The listing builds one solid part. Answer for the finished solid, in the listing's coordinates (mm). A direction names the side the tool comes from. Give positions to 0.01 mm unless a question says otherwise; leave off trailing zeros. Loops run counter-clockwise (first coordinate to the right, second up) from the corner with the lowest first, then second, coordinate; pieces in that order, holes last. Notation, with made-up numbers: M 57.25,19.25 L 68.25,19.25 A28 cw 68.25,57.25 Z; hole C 20.25,36.25 d7. An arc over 180 degrees is marked long. One line per item, written item: value. Start each with the question number.
Q1. A cutting plane is placed at D-D, the plane x = 47.5. Determine the outline of the cut face in (y, z), and give its area (3 significant figures).
Q2. Flat-ended cylindrical pins translate along their axes: pin 1 (8 mm diameter, centred on x = 54.5, y = 20, fed in from +Z); pin 2 (5 mm diameter, centred on x = 47.5, y = 15, fed in from +Z). Find the tip coordinate at first contact, or state that the pin passes through.
Q3. The mould has two halves that part along Y. Classify faces 1 (the flat face through (4.5, 5.7, 6)), 2 (the flat face through (32, 0, 1)), 3 (the cylindrical face through (4.109, 45.974, 4.479)), 4 (the cylindrical face through (59.763, 43.676, 2.958)): +Y half, -Y half, draft (parallel to the pull), parting line (faces both ways), or undercut.
Q4. A cutting plane is placed at A-A, the plane z = 5. Determine the outline of the cut face in (x, y).
Q5. A cutting plane is placed at C-C, the plane y = 43. Determine the outline of the cut face in (x, z).
Q6. For faces 5 (the cylindrical face through (58.29, 45.03, 4.48)), 6 (the flat face through (32, 25, 0)), determine the directions among +Z, -Z, +X, -X, +Y, -Y from which every point of the face is accessible in a straight line to the end or side of a thin tool.
Q7. A cutting plane is placed at B-B, the plane x = 4.5. Determine the outline of the cut face in (y, z).
Q8. Consider L1, parallel to Y at x = 60.5, z = 1.3; L2, parallel to Y at x = 4.5, z = 3.05; L3, parallel to Z at x = 36, y = 28.5. Determine where each line is inside the solid, lowest interval first.
from build123d import *

# Parameters (mm, degrees)
F0_W     = 65
F0_H     = 50
F0_R     = 1
F0_R_2   = 1.9
F1_DEPTH = 3
F2_SIZE  = 2
F3_R     = 3
F3_R_2   = 1
F4_DEPTH = 3


with BuildPart() as f1:
    # F0 (on Top) → F1 (new body)
    with BuildSketch(Plane.XY):
        with Locations((32.5, 25)):
            Rectangle(F0_W, F0_H)
        with Locations((4.5, 7)):
            Circle(F0_R, mode=Mode.SUBTRACT)
        with Locations((17.5, 15)):
            Circle(F0_R_2, mode=Mode.SUBTRACT)
        with Locations((60.5, 7)):
            Circle(F0_R, mode=Mode.SUBTRACT)
        with Locations((47.5, 15)):
            Circle(F0_R_2, mode=Mode.SUBTRACT)
        with Locations((4.5, 43)):
            Circle(F0_R, mode=Mode.SUBTRACT)
        with Locations((60.5, 43)):
            Circle(F0_R, mode=Mode.SUBTRACT)
    extrude(amount=F1_DEPTH)

    # F2
    f2_edges = [f1.edges().sort_by_distance(p)[0] for p in [
        (15.6, 15, 3),
        (45.6, 15, 3),
    ]]
    chamfer(f2_edges, length=F2_SIZE)

    # F3 (on face) → F4 (join)
    with BuildSketch(Plane.XY.offset(3)):
        with Locations((4.5, 43)):
            Circle(F3_R)
        with Locations((4.5, 43)):
            Circle(F3_R_2, mode=Mode.SUBTRACT)
        with Locations((60.5, 43)):
            Circle(F3_R)
        with Locations((60.5, 43)):
            Circle(F3_R_2, mode=Mode.SUBTRACT)
        with Locations((60.5, 7)):
            Circle(F3_R)
        with Locations((60.5, 7)):
            Circle(F3_R_2, mode=Mode.SUBTRACT)
        with Locations((4.5, 7)):
            Circle(F3_R)
        with Locations((4.5, 7)):
            Circle(F3_R_2, mode=Mode.SUBTRACT)
    extrude(amount=F4_DEPTH)


solid = f1.part
Answer block:
1. outline: M 0,0 L 13.1,0 L 13.1,1 L 11.1,3 L 0,3 Z; M 16.9,0 L 50,0 L 50,3 L 18.9,3 L 16.9,1 Z
1. area: 135 mm^2
2. pin 1: z = 3
2. pin 2: z = 1.6
3. face 1: draft
3. face 2: -Y half
3. face 3: undercut
3. face 4: undercut
4. outline: C 4.5,7 d6; C 4.5,43 d6; C 60.5,7 d6; C 60.5,43 d6; hole C 4.5,7 d2; hole C 4.5,43 d2; hole C 60.5,7 d2; hole C 60.5,43 d2
5. outline: M 0,0 L 3.5,0 L 3.5,6 L 1.5,6 L 1.5,3 L 0,3 Z; M 5.5,0 L 59.5,0 L 59.5,6 L 57.5,6 L 57.5,3 L 7.5,3 L 7.5,6 L 5.5,6 Z; M 61.5,0 L 65,0 L 65,3 L 63.5,3 L 63.5,6 L 61.5,6 Z
6. face 5: +Z
6. face 6: -Z, +X, -X, +Y, -Y
7. outline: M 0,0 L 6,0 L 6,6 L 4,6 L 4,3 L 0,3 Z; M 8,0 L 42,0 L 42,6 L 40,6 L 40,3 L 10,3 L 10,6 L 8,6 Z; M 44,0 L 50,0 L 50,3 L 46,3 L 46,6 L 44,6 Z
8. L1: 0 to 6, 8 to 42, 44 to 50
8. L2: 4 to 6, 8 to 10, 40 to 42, 44 to 46
8. L3: 0 to 3
